CAD build for the part. Positions are in the model's coordinates, mm. Face numbers are marked on the shaded views. A direction names the side the tool comes from. Round coordinates to 2 decimals unless told otherwise and drop trailing zeros. Write each loop counter-clockwise with the first axis right and the second up, starting at its lowest first coordinate (ties: lowest second). Pieces come first, ordered by that corner, then holes. Notation, with made-up numbers: (19.25, 60.5) - (29.25, 60.5) arc R14 ccw to (29.25, 64.5) - close; hole circle Ø4 at (1, 89). An arc over 180 degrees is marked (long way). Put each result on its own line as item: value. Start each with the question number.
Item 1: Mould opens along Z. For the marked faces 1, 2 and 3 say: released by +Z, released by -Z, zero draft, split by the parting line, or undercut.
Item 2: 3-axis set-ups, long thin cutter, end or side, ignore diameter. For the marked faces 4 and 5: which of +Z, -Z, +X, -X, +Y, -Y reach the whole face in a straight line?
Item 3: Cut at C-C (y = -0.5). Count the separate pieces of the cut face and the enclosed holes in it, and give its area (3 significant figures).
Item 4: Cut at B-B (z = -10.5). Give the cut face in (x, y).
Item 5: Cut at D-D (x = 3.5). Give the cut face in (y, z), and give its area (3 significant figures).
Item 6: Drill centre lines: line 1 (Z direction, x = -8.5, y = 0); line 2 (X direction, y = -0.75, z = 0.75); line 3 (Z direction, x = 7, y = 1.5). Where is each one in solid material? Low to high. Write a range as from..to.
Item 7: Pin check, flat tips, straight feed: pin 1 Ø1.5 at (x, y) = (-3.5, 0) entering from -Z; pin 2 Ø8.5 at (x, z) = (1, -0.5) entering from +Y; pin 3 Ø1 at (y, z) = (2, 3) entering from +X; pin 4 Ø1 at (x, y) = (-6, 0) entering from +Z. Stop position of each tip, or through.
Item 8: Cut at A-A (x = -11). Give the cut face in (y, z) (3 decimals), and give its area (3 significant figures).
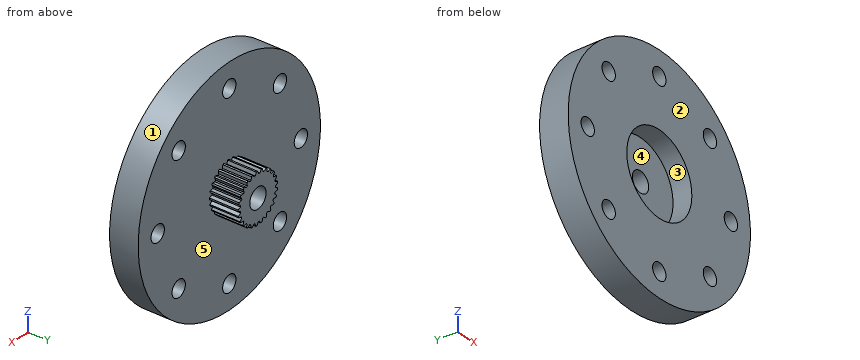
```python
from build123d import *

# Parameters (mm, degrees)
SKETCH1_R                          = 14
BOSS_EXTRUDE1_DEPTH                = 1.75
TAP_DRILL_FOR_M2_5X0_45_TAP1_D     = 2.05
TAP_DRILL_FOR_M2_5X0_45_TAP1_DEPTH = 6
TAP_DRILL_FOR_M2_5X0_45_TAP1_TIP   = 0.615882135
SKETCH7_R                          = 5
CUT_EXTRUDE1_DEPTH                 = 2.3
BOSS_EXTRUDE3_DEPTH                = 3.5
TAP_DRILL_FOR_M3X0_5_TAP1_D        = 2.5
TAP_DRILL_FOR_M3X0_5_TAP1_DEPTH    = 6
TAP_DRILL_FOR_M3X0_5_TAP1_TIP      = 0.751075774


with BuildPart() as part:
    # Sketch1 → Boss-Extrude1 (new, symmetric)
    with BuildSketch(Plane(origin=(0, 0, 0), x_dir=(1, 0, 0), z_dir=(0, 1, 0))):
        with Locations(Location((0, 0, 0), (0, 0, 270))):
            Circle(SKETCH1_R)
    extrude(amount=BOSS_EXTRUDE1_DEPTH, both=True)

    # Tap Drill for M2.5x0.45 Tap1
    with Locations(Plane(origin=(0, 1.75, 0), x_dir=(1, 0, 0), z_dir=(0, 1, 0))):
        with Locations((-11, 0), (-7.778174593, 7.778174593), (0, 11), (7.778174593, 7.778174593), (11, 0), (7.778174593, -7.778174593), (0, -11), (-7.778174593, -7.778174593)):
            Hole(TAP_DRILL_FOR_M2_5X0_45_TAP1_D / 2, depth=TAP_DRILL_FOR_M2_5X0_45_TAP1_DEPTH)
            with Locations((0, 0, -(TAP_DRILL_FOR_M2_5X0_45_TAP1_DEPTH + TAP_DRILL_FOR_M2_5X0_45_TAP1_TIP / 2))):  # 118° drill point
                Cone(0, TAP_DRILL_FOR_M2_5X0_45_TAP1_D / 2, TAP_DRILL_FOR_M2_5X0_45_TAP1_TIP, mode=Mode.SUBTRACT)

    # Sketch7 → Cut-Extrude1 (cut)
    with BuildSketch(Plane.XZ.offset(1.75)):
        with Locations(Location((0, 0, 0), (0, 0, 270))):
            Circle(SKETCH7_R)
    extrude(amount=-CUT_EXTRUDE1_DEPTH, mode=Mode.SUBTRACT)

    # Sketch8 → Boss-Extrude3 (add)
    with BuildSketch(Plane(origin=(0, 1.75, 0), x_dir=(1, 0, 0), z_dir=(0, 1, 0))):
        with BuildLine():
            Line((-0.128852443, -2.696923627), (0.057352661, -3.049460718))
            ThreePointArc((0.057352661, -3.049460718), (0.151245078, -3.04624768), (0.244993995, -3.040144395))
            Line((0.244993995, -3.040144395), (0.395362741, -2.670896535))
            ThreePointArc((0.395362741, -2.670896535), (0.470816738, -2.658633408), (0.545893326, -2.644239111))
            Line((0.545893326, -2.644239111), (0.813920864, -2.939393275))
            ThreePointArc((0.813920864, -2.939393275), (0.904064427, -2.912931086), (0.993350224, -2.883705139))
            Line((0.993350224, -2.883705139), (1.047166652, -2.488662694))
            ThreePointArc((1.047166652, -2.488662694), (1.117200406, -2.458020189), (1.18633861, -2.425407327))
            Line((1.18633861, -2.425407327), (1.519347425, -2.644632943))
            ThreePointArc((1.519347425, -2.644632943), (1.600078084, -2.596584319), (1.679290606, -2.546072084))
            Line((1.679290606, -2.546072084), (1.63317323, -2.150057022))
            ThreePointArc((1.63317323, -2.150057022), (1.693386265, -2.102960522), (1.752241875, -2.054178281))
            Line((1.752241875, -2.054178281), (2.1293078, -2.183700596))
            ThreePointArc((2.1293078, -2.183700596), (2.19555295, -2.11708461), (2.259714983, -2.048459957))
            Line((2.259714983, -2.048459957), (2.116561528, -1.676355361))
            ThreePointArc((2.116561528, -1.676355361), (2.163170436, -1.615764111), (2.208045339, -1.553877659))
            Line((2.208045339, -1.553877659), (2.605475935, -1.58555831))
            ThreePointArc((2.605475935, -1.58555831), (2.653073149, -1.504560688), (2.698153157, -1.422135556))
            Line((2.698153157, -1.422135556), (2.466958481, -1.097322127))
            ThreePointArc((2.466958481, -1.097322127), (2.497034654, -1.027043299), (2.525109194, -0.955941189))
            Line((2.525109194, -0.955941189), (2.917932434, -0.887789563))
            ThreePointArc((2.917932434, -0.887789563), (2.943891005, -0.797499685), (2.967056445, -0.706453148))
            Line((2.967056445, -0.706453148), (2.66234736, -0.449340108))
            ThreePointArc((2.66234736, -0.449340108), (2.674001, -0.373789578), (2.683511152, -0.297939418))
            Line((2.683511152, -0.297939418), (3.047044507, -0.134237734))
            ThreePointArc((3.047044507, -0.134237734), (3.049733363, -0.040328844), (3.049528665, 0.053618309))
            Line((3.049528665, 0.053618309), (2.690451163, 0.226875602))
            ThreePointArc((2.690451163, 0.226875602), (2.68295003, 0.302950716), (2.673298235, 0.378782983))
            Line((2.673298235, 0.378782983), (2.984699568, 0.627748746))
            ThreePointArc((2.984699568, 0.627748746), (2.963949757, 0.719376006), (2.940387783, 0.810320731))
            Line((2.940387783, 0.810320731), (2.549504025, 0.888835884))
            ThreePointArc((2.549504025, 0.888835884), (2.523319442, 0.960655502), (2.495112158, 1.031705055))
            Line((2.495112158, 1.031705055), (2.734814978, 1.350291464))
            ThreePointArc((2.734814978, 1.350291464), (2.691930287, 1.433879817), (2.646491522, 1.516107721))
            Line((2.646491522, 1.516107721), (2.248362172, 1.494947338))
            ThreePointArc((2.248362172, 1.494947338), (2.205139413, 1.55799877), (2.160149007, 1.619801305))
            Line((2.160149007, 1.619801305), (2.313091905, 1.987990402))
            ThreePointArc((2.313091905, 1.987990402), (2.250766937, 2.058287685), (2.186306467, 2.126632087))
            Line((2.186306467, 2.126632087), (1.805947455, 2.007125753))
            ThreePointArc((1.805947455, 2.007125753), (1.748402365, 2.057447246), (1.68945575, 2.106119481))
            Line((1.68945575, 2.106119481), (1.74602876, 2.500776593))
            ThreePointArc((1.74602876, 2.500776593), (1.668179623, 2.553365768), (1.588747735, 2.603532338))
            Line((1.588747735, 2.603532338), (1.250058417, 2.393189076))
            ThreePointArc((1.250058417, 2.393189076), (1.181806766, 2.427618744), (1.112607775, 2.460102424))
            Line((1.112607775, 2.460102424), (1.069256207, 2.856429793))
            ThreePointArc((1.069256207, 2.856429793), (0.980774447, 2.888006489), (0.89136214, 2.916843077))
            Line((0.89136214, 2.916843077), (0.615623612, 2.628879527))
            ThreePointArc((0.615623612, 2.628879527), (0.540953902, 2.645254028), (0.465850562, 2.659508085))
            Line((0.465850562, 2.659508085), (0.325298354, 3.032603004))
            ThreePointArc((0.325298354, 3.032603004), (0.231743607, 3.041183141), (0.137968984, 3.046877838))
            Line((0.137968984, 3.046877838), (-0.057493089, 2.699387809))
            ThreePointArc((-0.057493089, 2.699387809), (-0.133889085, 2.696678274), (-0.210177756, 2.691807071))
            Line((-0.210177756, 2.691807071), (-0.439099191, 3.018226615))
            ThreePointArc((-0.439099191, 3.018226615), (-0.531848537, 3.003271072), (-0.624093271, 2.985466059))
            Line((-0.624093271, 2.985466059), (-0.726997287, 2.600283627))
            ThreePointArc((-0.726997287, 2.600283627), (-0.800319329, 2.578660305), (-0.872999832, 2.55496992))
            Line((-0.872999832, 2.55496992), (-1.175906519, 2.814203948))
            ThreePointArc((-1.175906519, 2.814203948), (-1.262022681, 2.776652436), (-1.346941451, 2.736466467))
            Line((-1.346941451, 2.736466467), (-1.350821572, 2.337794062))
            ThreePointArc((-1.350821572, 2.337794062), (-1.416462566, 2.298615626), (-1.480968118, 2.257594612))
            Line((-1.480968118, 2.257594612), (-1.838827315, 2.433354496))
            ThreePointArc((-1.838827315, 2.433354496), (-1.912899299, 2.375566516), (-1.985156345, 2.315524624))
            Line((-1.985156345, 2.315524624), (-1.88976877, 1.928412299))
            ThreePointArc((-1.88976877, 1.928412299), (-1.943604251, 1.874140474), (-1.995881731, 1.818366332))
            Line((-1.995881731, 1.818366332), (-2.386207829, 1.899608433))
            ThreePointArc((-2.386207829, 1.899608433), (-2.443581419, 1.825215014), (-2.498636566, 1.749089852))
            Line((-2.498636566, 1.749089852), (-2.309974846, 1.397861298))
            ThreePointArc((-2.309974846, 1.397861298), (-2.348622132, 1.331906183), (-2.385386754, 1.264883407))
            Line((-2.385386754, 1.264883407), (-2.783654129, 1.246502985))
            ThreePointArc((-2.783654129, 1.246502985), (-2.820724331, 1.160178541), (-2.855118261, 1.072753333))
            Line((-2.855118261, 1.072753333), (-2.585036707, 0.779477531))
            ThreePointArc((-2.585036707, 0.779477531), (-2.606067447, 0.705983328), (-2.625009154, 0.631923206))
            Line((-2.625009154, 0.631923206), (-3.006193202, 0.51507517))
            ThreePointArc((-3.006193202, 0.51507517), (-3.02063076, 0.422243783), (-3.032202376, 0.329011776))
            Line((-3.032202376, 0.329011776), (-2.697671205, 0.112116324))
            ThreePointArc((-2.697671205, 0.112116324), (-2.69976396, 0.035700944), (-2.699692576, -0.040743054))
            Line((-2.699692576, -0.040743054), (-3.0398421, -0.248716711))
            ThreePointArc((-3.0398421, -0.248716711), (-3.030739849, -0.342222105), (-3.018762064, -0.435402801))
            Line((-3.018762064, -0.435402801), (-2.640801099, -0.562289564))
            ThreePointArc((-2.640801099, -0.562289564), (-2.623824375, -0.636824661), (-2.604744383, -0.710849278))
            Line((-2.604744383, -0.710849278), (-2.88248654, -0.996880808))
            ThreePointArc((-2.88248654, -0.996880808), (-2.850416406, -1.085184919), (-2.815641829, -1.172459418))
            Line((-2.815641829, -1.172459418), (-2.417999748, -1.201364731))
            ThreePointArc((-2.417999748, -1.201364731), (-2.383020254, -1.269336231), (-2.346130522, -1.336290227))
            Line((-2.346130522, -1.336290227), (-2.544013749, -1.682407216))
            ThreePointArc((-2.544013749, -1.682407216), (-2.490990819, -1.759961574), (-2.435604463, -1.835846099))
            Line((-2.435604463, -1.835846099), (-2.04326658, -1.764953733))
            ThreePointArc((-2.04326658, -1.764953733), (-1.992482207, -1.822090738), (-1.940100652, -1.877767147))
            Line((-1.940100652, -1.877767147), (-2.045691219, -2.262221792))
            ThreePointArc((-2.045691219, -2.262221792), (-1.975047116, -2.32415337), (-1.902529111, -2.383879817))
            Line((-1.902529111, -2.383879817), (-1.540147459, -2.217644202))
            ThreePointArc((-1.540147459, -2.217644202), (-1.476749174, -2.260356582), (-1.412167122, -2.301257052))
            Line((-1.412167122, -2.301257052), (-1.418830385, -2.699892653))
            ThreePointArc((-1.418830385, -2.699892653), (-1.33500394, -2.742310063), (-1.249910858, -2.782125599))
            Line((-1.249910858, -2.782125599), (-0.940255208, -2.530991929))
            ThreePointArc((-0.940255208, -2.530991929), (-0.86822656, -2.556595909), (-0.795501939, -2.580150512))
            Line((-0.795501939, -2.580150512), (-0.70281922, -2.967919329))
            ThreePointArc((-0.70281922, -2.967919329), (-0.611077556, -2.988157329), (-0.518756109, -3.005560197))
            Line((-0.518756109, -3.005560197), (-0.281283264, -2.685308125))
            ThreePointArc((-0.281283264, -2.685308125), (-0.205150078, -2.692194912), (-0.128852443, -2.696923627))
        make_face()
    extrude(amount=BOSS_EXTRUDE3_DEPTH)

    # Tap Drill for M3x0.5 Tap1
    with Locations(Plane(origin=(0, 5.25, 0), x_dir=(1, 0, 0), z_dir=(0, 1, 0))):
        with Locations((0, 0)):
            Hole(TAP_DRILL_FOR_M3X0_5_TAP1_D / 2, depth=TAP_DRILL_FOR_M3X0_5_TAP1_DEPTH)
            with Locations((0, 0, -(TAP_DRILL_FOR_M3X0_5_TAP1_DEPTH + TAP_DRILL_FOR_M3X0_5_TAP1_TIP / 2))):  # 118° drill point
                Cone(0, TAP_DRILL_FOR_M3X0_5_TAP1_D / 2, TAP_DRILL_FOR_M3X0_5_TAP1_TIP, mode=Mode.SUBTRACT)


solid = part.part
```
Output values:
1. face 1: split by the parting line
1. face 2: zero draft
1. face 3: undercut
2. face 4: -Y
2. face 5: +Y
3. separate pieces: 1
3. enclosed holes: 9
3. area: 511 mm2
4. outline: (-9.26, -1.75) - (-0.89, -1.75) - (-0.89, 1.75) - (-9.26, 1.75) - close; (0.89, -1.75) - (9.26, -1.75) - (9.26, 1.75) - (0.89, 1.75) - close
5. outline: (-1.75, -13.56) - (1.75, -13.56) - (1.75, 13.56) - (-1.75, 13.56) - (-1.75, 3.57) - (0.55, 3.57) - (0.55, -3.57) - (-1.75, -3.57) - close
5. area: 78.5 mm2
6. line 1: -11.12..-8.51, -7.05..7.05, 8.51..11.12
6. line 2: -13.98..-11.7, -10.3..-4.94, 4.94..10.3, 11.7..13.98
6. line 3: -12.12..-8.45, -7.11..7.11, 8.45..12.12
7. pin 1: z = -13.73
7. pin 2: y = 5.25
7. pin 3: x = 13.76
7. pin 4: z = 12.87
8. outline: (-1.75, -8.66) - (1.75, -8.66) - (1.75, -1.025) - (-1.75, -1.025) - close; (-1.75, 1.025) - (1.75, 1.025) - (1.75, 8.66) - (-1.75, 8.66) - close
8. area: 53.4 mm2
